The drawing under review shows one solid part. Ordinate dimensions are in mm from its lowest x, y, z. A direction names the side the tool comes from. Coordinates: 2 decimals unless noted, no trailing zeros. Write each loop counter-clockwise with the first axis right and the second up, starting at its lowest first coordinate (ties: lowest second). Pieces come first, ordered by that corner, then holes.
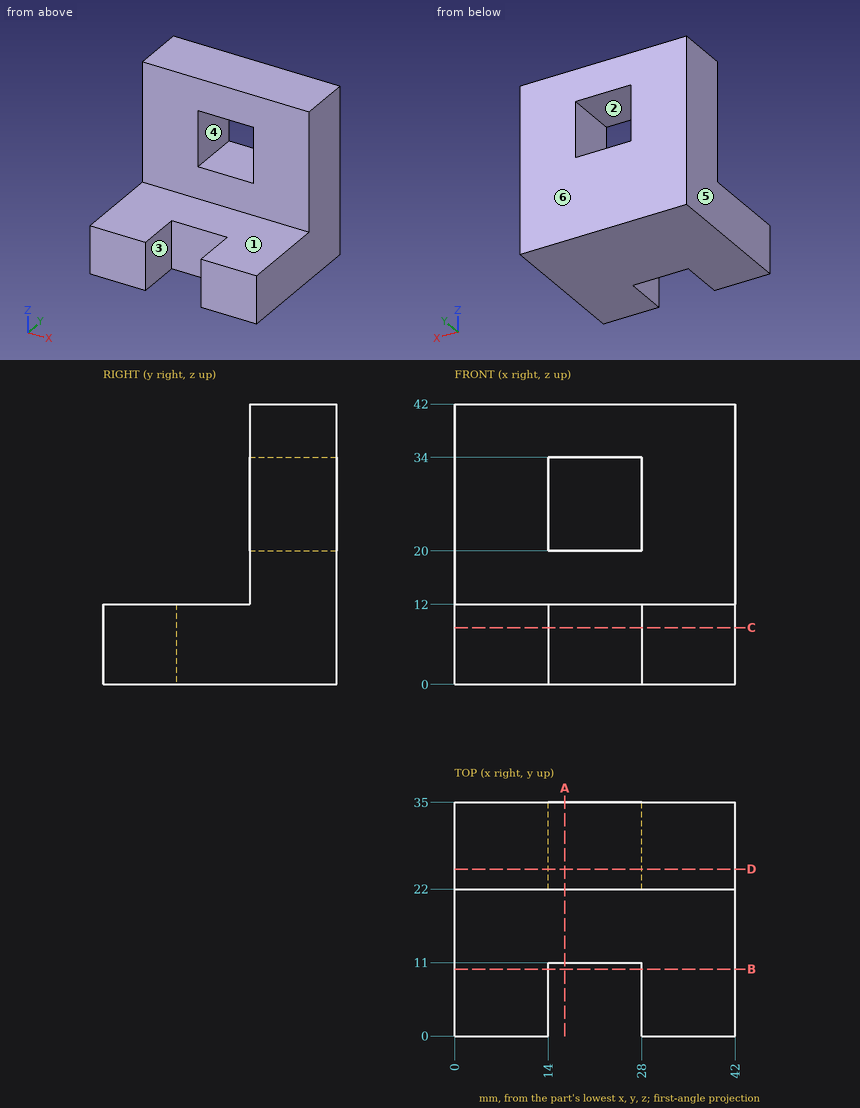
Q1. Tool access review of the marked faces 1, 2 and 3: name each direction out of +Z, -Z, +X, -X, +Y, -Y from which nothing blocks a thin tool from reaching the whole face with its end or side.
Ans:
face 1: +Z, +X, -X, -Y
face 2: +Y, -Y
face 3: +Z, -Z, -Y
Q2. Add section A-A (x = 16.5). State the section outline as (y, z) points, then the cut area to 3 significant figures.
Ans:
outline: (11, 0) - (35, 0) - (35, 20) - (22, 20) - (22, 12) - (11, 12) - close; (22, 34) - (35, 34) - (35, 42) - (22, 42) - close
area: 496 mm2
Q3. Draft analysis for pull direction X (two halves, no side actions). For the marked faces 4, 5 and 6, state which applies: +X half, -X half, draft (parallel to the pull), parting line (faces both ways), or undercut.
Ans:
face 4: undercut
face 5: -X half
face 6: draft
Q4. For probe 1 along X at (y, z) = (33, 24); probe 2 along Z at (x, y) = (24, 29); probe 3 along Y at (x, z) = (29, 20), list the stretches that pass through material, from the lowest coordinate up.
Ans:
probe 1: x = 0 to 14, 28 to 42
probe 2: z = 0 to 20, 34 to 42
probe 3: y = 22 to 35
Q5. Add section D-D (y = 25). State the section outline as (x, z) points.
Ans:
outline: (0, 0) - (42, 0) - (42, 42) - (0, 42) - close; hole (14, 20) - (28, 20) - (28, 34) - (14, 34) - close
Q6. Add section B-B (y = 10). State the section outline as (x, z) points.
Ans:
outline: (0, 0) - (14, 0) - (14, 12) - (0, 12) - close; (28, 0) - (42, 0) - (42, 12) - (28, 12) - close
Q7. Clearance check with flat-ended pins moving along their axes: pin 1 Ø3 at (x, z) = (9, 30.5) entering from -Y; pin 2 Ø3.5 at (x, z) = (23, 5) entering from -Y; pin 3 Ø1 at (y, z) = (20.5, 29) entering from -X. State where each tip first meets the part, or that it passes through.
Ans:
pin 1: stops at y = 22
pin 2: stops at y = 11
pin 3: passes through
Q8. Add section C-C (z = 8.5). State the section outline as (x, y) points, then the cut area to 3 significant figures.
Ans:
outline: (0, 0) - (14, 0) - (14, 11) - (28, 11) - (28, 0) - (42, 0) - (42, 35) - (0, 35) - close
area: 1,320 mm2
